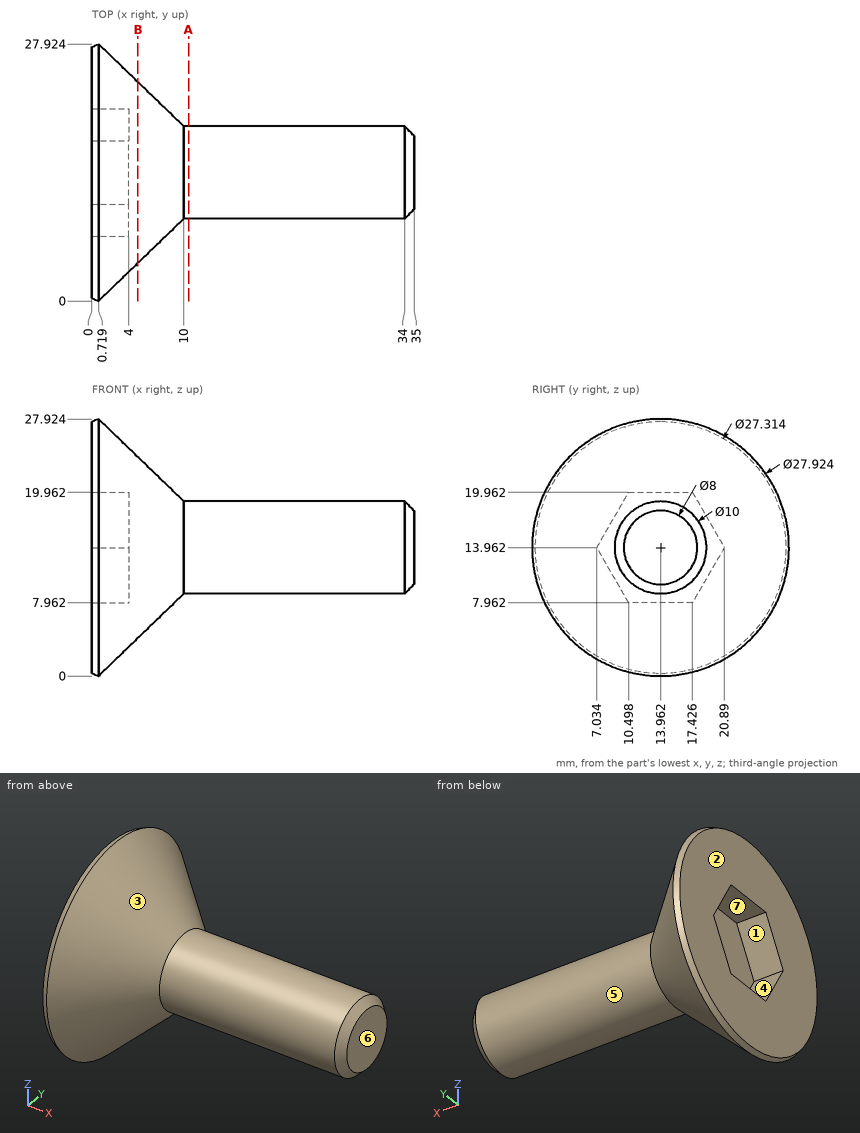
Could you check a few things on this drawing? It's one solid part, dimensions in mm from its lowest x, y, z. A direction names the side the tool comes from. Coordinates: 2 decimals unless noted, no trailing zeros. Order: outer loops, then holes, each group sorted by start corner. A loop starts at its lowest first (then second) coordinate and runs counter-clockwise, first axis right, second up. Notation, with made-up numbers: M 15.25,-17 L 35.25,-17 A12 cw 35.25,-7 Z; hole C -27,0 d3. An arc over 180 degrees is marked long. Answer as a JSON object with one key per item and string values. Group by question number.
(1) Suppose I cut it at A-A, the plane x = 10.5. Please give me the cut outline in (y, z).
(2) For pin 1 (8 mm diameter, centred on x = 26.5, z = 18, fed in from +Y); pin 2 (1.5 mm diameter, centred on x = 4.5, z = 13, fed in from -Y) (1 decimal); pin 3 (1.5 mm diameter, centred on x = 29.5, z = 7.5, fed in from +Y); pin 4 (1 mm diameter, centred on y = 6.5, z = 24, fed in from +X) (1 decimal), each with a flat end and sliding along its axis, tell me the tip position at first contact or that it passes through.
(3) Which directions (+Z, -Z, +X, -X, +Y, -Y) give clear straight access to the entire face, cutting with the end or side of a thin tool? Please do the marked faces 5, 6 and 7.
(4) I need wall thicknesses on probe 1 along X at (y, z) = (12.75, 13.75); probe 2 along X at (y, z) = (11, 22) (1 decimal); probe 3 along Y at (x, z) = (18.5, 14.5). Which ranges of each line are inside material? Lowest first, please.
(5) If we mould it in two halves opening along Y, with no side actions, what happens to the marked faces 1, 2, 3 and 4? For each: released by +Y, released by -Y, zero draft, split by the parting line, or undercut.
(6) Suppose I cut it at B-B, the plane x = 5. Please give me the cut outline in (y, z).
Values found:
{
 "1": {"outline": "C 13.96,13.96 d10"},
 "2": {"pin 1": "stops at y = 18.96", "pin 2": "stops at y = 3", "pin 3": "passes through", "pin 4": "stops at x = 2.7"},
 "3": {"face 5": "+X", "face 6": "+Z, -Z, +X, +Y, -Y", "face 7": "-X"},
 "4": {"probe 1": "x = 4 to 35", "probe 2": "x = 0 to 6.3", "probe 3": "y = 8.99 to 18.93"},
 "5": {"face 1": "undercut", "face 2": "zero draft", "face 3": "split by the parting line", "face 4": "undercut"},
 "6": {"outline": "C 13.96,13.96 d19.66"}
}
